For this review, take the finished solid that the model builds, in its own axes (mm). A direction names the side the tool comes from. Round coordinates to 2 decimals unless told otherwise and drop trailing zeros. Order: outer loops, then holes, each group sorted by start corner. A loop starts at its lowest first (then second) coordinate and runs counter-clockwise, first axis right, second up. Notation, with made-up numbers: (64.5, 7.5) - (102.5, 7.5) arc R24 cw to (102.5, 42.5) - close; hole circle Ø11 at (87.5, 50). An arc over 180 degrees is marked (long way). One line per item, written item: value.
```python
from build123d import *

# Parameters (mm, degrees)
SKETCH1_R           = 56.515
BOSS_EXTRUDE1_DEPTH = 12.7
CHAMFER1_SIZE       = 1.27
SKETCH2_R           = 50.165
BOSS_EXTRUDE2_DEPTH = 3.175
CHAMFER2_SIZE       = 1.27
SKETCH3_R           = 3.175
CUT_EXTRUDE1_DEPTH  = 16.875


with BuildPart() as part:
    # Sketch1 → Boss-Extrude1 (new body)
    with BuildSketch(Plane(origin=(0, 0, 0), x_dir=(1, 0, 0), z_dir=(0, 1, 0))):
        Circle(SKETCH1_R)
    extrude(amount=BOSS_EXTRUDE1_DEPTH)

    # Chamfer1
    chamfer1_edges = [part.edges().sort_by_distance(p)[0] for p in [
        (-56.515, 0, 0),
        (-56.515, 12.7, 0),
    ]]
    chamfer(chamfer1_edges, length=CHAMFER1_SIZE)

    # Sketch2 → Boss-Extrude2 (add)
    with BuildSketch(Plane.XZ):
        Circle(SKETCH2_R)
    extrude(amount=BOSS_EXTRUDE2_DEPTH)

    # Chamfer2
    chamfer2_edges = [part.edges().sort_by_distance(p)[0] for p in [
        (-50.165, -3.175, 0),
    ]]
    chamfer(chamfer2_edges, length=CHAMFER2_SIZE)

    # Sketch3 → Cut-Extrude1 (cut, through all)
    with BuildSketch(Plane(origin=(0, 12.7, 0), x_dir=(1, 0, 0), z_dir=(0, 1, 0))):
        with Locations((-38.1, 0)):
            Circle(SKETCH3_R)
        with Locations((38.1, 0)):
            Circle(SKETCH3_R)
    extrude(amount=-CUT_EXTRUDE1_DEPTH, mode=Mode.SUBTRACT)


solid = part.part
```
Item 1: Machinability: for faces 4 (the flat face through (-1, 12.7, -1)), 5 (the flat face through (12, 0, 49)), which of the approach directions +Z, -Z, +X, -X, +Y, -Y give a long, thin tool a straight path to every point of the face, cutting with its end or side? Answer none if there is none.
Returned:
face 4: +Z, -Z, +X, -X, +Y
face 5: -Y
Item 2: Take a section at B-B (x = 0). Write out the cut boundary in (y, z) (3 decimals).
Returned:
outline: (-3.175, -48.895) - (-1.905, -50.165) - (0, -50.165) - (0, -55.245) - (1.27, -56.515) - (11.43, -56.515) - (12.7, -55.245) - (12.7, 55.245) - (11.43, 56.515) - (1.27, 56.515) - (0, 55.245) - (0, 50.165) - (-1.905, 50.165) - (-3.175, 48.895) - close
Item 3: Wall thickness on line 1 (X direction, y = 8.75, z = 0) (3 decimals); line 2 (Z direction, x = -38.1, y = 8.5) (3 decimals); line 3 (Z direction, x = 0, y = 5.5) (3 decimals): over which ranges is each line inside the solid? List them lowest first.
Returned:
line 1: -56.515 to -41.275, -34.925 to 34.925, 41.275 to 56.515
line 2: -41.741 to -3.175, 3.175 to 41.741
line 3: -56.515 to 56.515
Item 4: For P1, Ø4, axis at y = 4.5, z = -11.5, coming from the +X side; P2, Ø1.5, axis at y = -1, z = -35.5, coming from the -X side; P3, Ø8, axis at y = 0.5, z = 34, coming from the -X side, all flat-tipped, find the tip position at first contact; note any pin that passes through.
Returned:
P1: x = 55.71
P2: x = -36.18
P3: x = -47.85
Item 5: Take a section at C-C (y = 4). Write out the cut boundary in (x, z) (3 decimals).
Returned:
outline: circle Ø113.03 at (0, 0); hole circle Ø6.35 at (-38.1, 0); hole circle Ø6.35 at (38.1, 0)
Item 6: Take a section at A-A (z = 0). Write out the cut boundary in (x, y) (3 decimals), plus the area to 3 significant figures.
Returned:
outline: (-56.515, 1.27) - (-55.245, 0) - (-50.165, 0) - (-50.165, -1.905) - (-48.895, -3.175) - (-41.275, -3.175) - (-41.275, 12.7) - (-55.245, 12.7) - (-56.515, 11.43) - close; (-34.925, -3.175) - (34.925, -3.175) - (34.925, 12.7) - (-34.925, 12.7) - close; (41.275, -3.175) - (48.895, -3.175) - (50.165, -1.905) - (50.165, 0) - (55.245, 0) - (56.515, 1.27) - (56.515, 11.43) - (55.245, 12.7) - (41.275, 12.7) - close
area: 1,550 mm^2
Item 7: The part is to be moulded in two halves that separate along Z. For faces 1 (the flat face through (-1, -3.175, 1)), 2 (the cylindrical face through (-41.27, 4.87, -0.14)), 3 (the cylindrical face through (-6.53, -0.94, 49.74)), say which applies: +Z half, -Z half, draft (parallel to the pull), parting line (faces both ways), or undercut.
Returned:
face 1: draft
face 2: undercut
face 3: parting line
